Input: part model. Units: mm. Frame: model coordinates. A direction names the side the tool comes from. Round coordinates to 2 decimals unless told otherwise and drop trailing zeros. Loops run counter-clockwise (first coordinate to the right, second up) from the corner with the lowest first, then second, coordinate; pieces in that order, holes last. Notation, with made-up numbers: (2, 54.25) -> (29, 54.25) arc R22 cw to (29, 92.25) -> close; hole circle Ø1 at (-1.5, 75.5). An arc over 180 degrees is marked (long way). Answer as a JSON object with one key per item and string values.
Autodesk Inventor part; units mm, degrees
ref_plane "YZ Plane" through (0, 0, 0) normal (1, 0, 0) x (0, 1, 0)
ref_plane "XZ Plane" through (0, 0, 0) normal (0, 1, 0) x (-1, 0, 0)
ref_plane "XY Plane" through (0, 0, 0) normal (0, 0, 1) x (1, 0, 0)
sketch "Sketch1" plane through (0, 0, 0) normal (0, 0, 1) x (1, 0, 0)
  circle A0 centre (0, 0) radius 3
  dimension "d0" = 6
extrude "Extrusion1" add sketch "Sketch1" along normal blind 34.05
sketch "Sketch2" plane through (0, 0, 34.05) normal (0, 0, 1) x (1, 0, 0)
  circle A0 centre (0, 0) radius 2
  dimension "d3" = 4
hole "Hole1" at (0, 0, 34.05) direction (0, 0, -1) diameter 2.459 depth 8.8 tip angle 118
chamfer "Chamfer1" distance 0.3 angle 45 1 edges at (0, 1.2295, 34.05)
sketch "Sketch3" plane through (0, 0, 34.05) normal (0, 0, 1) x (1, 0, 0)
  circle A0 centre (0, 0) radius 3
  circle A1 centre (0, 0) radius 2.5
  dimension "d14" = 5
extrude "Extrusion2" cut sketch "Sketch3" against normal blind 1
sketch "Sketch4" plane through (0, 0, 0) normal (0, 0, -1) x (-1, 0, 0)
  circle A0 centre (0, 0) radius 1.5
  dimension "d17" = 3
extrude "Extrusion3" add sketch "Sketch4" along normal blind 1
sketch "Sketch5" plane through (0, 0, -1) normal (0, 0, -1) x (-1, 0, 0)
  point P0 (0, 0)
  point P1 (0, 0)
hole "Hole2" at (0, 0, -1) direction (0, 0, 1) diameter 2 depth 2.5 tip angle 118
ref_plane "Work Plane2" through (0, 0, -0.5) normal (0, 0, -1) x (-1, 0, 0)
sketch "Sketch7" plane through (0, 0, -0.5) normal (0, 0, -1) x (-1, 0, 0)
  circle A0 centre (0, 0) radius 1.4
  circle A1 centre (0, 0) radius 1.5
  dimension "d29" = 2.8
  dimension "d30" = 3
extrude "Extrusion4" cut sketch "Sketch7" against normal blind 0.5
sketch "Sketch8" plane through (0, 0, 33.05) normal (0, 0, 1) x (1, 0, 0)
  circle A0 centre (0, 0) radius 2.5
  circle A1 centre (0, 0) radius 2.5
  circle A2 centre (0, 0) radius 2.3
  dimension "d31" = 4.6
extrude "Extrusion5" cut sketch "Sketch8" along normal blind 0.2
chamfer "Chamfer2" distance 0.2 angle 45 2 edges at (1.5, 0, -1) (-2.5, 0, 34.05)
properties part number "słupek"
1) Draft query along Y for faces 5 (the face through (0.748, 0.976, 29.44)), 6 (the face through (0, -2, 34.05)), 7 (the face through (-0.21, 0.05, 24.64)), 8 (the face through (1.4, 0.06, -0.25)). Return one class per face: +Y half, -Y half, draft (parallel to the pull), parting line (faces both ways), or undercut.
Output:
{"face 5": "undercut", "face 6": "draft", "face 7": "undercut", "face 8": "parting line"}
2) Ray query, probe 1 along Y at (x, z) = (0, 0.5); probe 2 along Y at (x, z) = (0, 27); probe 3 along Z at (x, y) = (-1.35, -2.6). Return the intervals inside material, ascending.
Output:
{"probe 1": "y = -3 to -1, 1 to 3", "probe 2": "y = -3 to -1.23, 1.23 to 3", "probe 3": "z = 0 to 33.05"}
3) Section A-A, the plane z = 32.5. Output: boundary loops of the cut face in (x, y).
Output:
{"outline": "circle Ø6 at (0, 0); hole circle Ø2.46 at (0, 0)"}
4) Section B-B, the plane z = 22.5. Output: boundary loops of the cut face in (x, y).
Output:
{"outline": "circle Ø6 at (0, 0)"}
5) Reachability of faces 1 (the face through (-0.54, -2.44, 33.55)), 2 (the face through (1, 0, 0)), 3 (the face through (2, -2, 33.05)), 4 (the face through (-3, 0, 16)) from +Z, -Z, +X, -X, +Y, -Y: full face, straight path, thin tool, end or side. Return the list, or none.
Output:
{"face 1": "+Z", "face 2": "-Z", "face 3": "none", "face 4": "+Z, -Z"}
6) Contact query for flat-ended pins moving along their axis: P1, Ø1, axis at x = -1, y = 2, coming from the -Z side; P2, Ø1.6, axis at x = 0, y = 0, coming from the +Z side; P3, Ø1.5, axis at x = 1, z = 10.5, coming from the -Y side. Output: stop coordinate, or through.
Output:
{"P1": "stops at z = 0", "P2": "stops at z = 24.99", "P3": "stops at y = -2.99"}
